Design review of the part built by this model. Coordinates are the model's own, in mm. A direction names the side the tool comes from. Round coordinates to 2 decimals unless told otherwise and drop trailing zeros. Loops run counter-clockwise (first coordinate to the right, second up) from the corner with the lowest first, then second, coordinate; pieces in that order, holes last. Notation, with made-up numbers: (-0.75, 2) - (45.25, 2) arc R21 ccw to (45.25, 40) - close; hole circle Ø4 at (23, 19.5). An arc over 180 degrees is marked (long way). Return JSON: item names as keys, results as strings. Group by question number.
(1) We need section D-D, the plane x = 20.5. Write out the cut boundary in (y, z).
(2) Clearance check with flat-ended pins moving along their axes: pin 1 (2 mm diameter, centred on x = -41.5, y = 46, fed in from +Z); pin 2 (1 mm diameter, centred on y = 9.5, z = 18.5, fed in from -X); pin 3 (0.6 mm diameter, centred on y = 21, z = 18.5, fed in from -X). State where each tip first meets the part, or that it passes through.
(3) We need section C-C, the plane x = -4. Write out the cut boundary in (y, z), and give its area (3 significant figures).
(4) We need section A-A, the plane z = 0. Write out the cut boundary in (x, y).
(5) The part is to be moulded in two halves that separate along Y. For faces 4 (the flat face through (-6, 85, 0)), 5 (the flat face through (-7, 83, 1)), 6 (the flat face through (-15, 42, -19.3)), 7 (the flat face through (3.201, 23, 18)), say which applies: pulls with the +Y half, pulls with the -Y half, needs draft (parallel to the pull), parting line crosses it, or undercut.
(6) We need section B-B, the plane y = 19. Write out the cut boundary in (x, z), and give its area (3 significant figures).
(7) For faces 1 (the cylindrical face through (30.597, 40.919, -0.383)), 2 (the flat face through (-40.799, 41, 0)), 3 (the flat face through (-2, 13, 18)), list the 3-axis set-ups (+Z, -Z, +X, -X, +Y, -Y) from which the entire face can be reached by the end or side of a thin tool; tool diameter is ignored.
(8) Wall thickness on L1, parallel to Y at x = 27, z = -1.5; L2, parallel to Z at x = 4.5, y = 19; L3, parallel to X at y = 32, z = 0.5: over which ranges is each line inside the solid? List them lowest first. Write a range as [from, to].
Autodesk Inventor part; units mm, degrees
ref_plane "Work Plane1" through (0, 85, 0) normal (0, 1, 0) x (1, 0, 0)
ref_plane "Work Plane2" through (-42.6987, 0, 19.3) normal (0, -1, 0) x (1, 0, 0)
ref_plane "YZ Plane" through (0, 0, 0) normal (1, 0, 0) x (0, 1, 0)
sketch "Sketch1" plane through (0, 0, 0) normal (0, 1, 0) x (-1, 0, 0)
  line L0 (40.7987, 17.4) -> (40.7987, -17.4)
  line L1 (40.7987, -17.4) -> (-13.2013, -17.4)
  arc A0 (-13.2013, 17.4) -> (-13.2013, -17.4) centre (-13.2013, 0) ccw
  line L2 (-13.2013, 17.4) -> (40.7987, 17.4)
  line L3 (42.6987, -19.3) -> (42.6987, 19.3)
  line L4 (42.6987, 19.3) -> (-13.2013, 19.3)
  arc A1 (-13.2013, 19.3) -> (-13.2013, -19.3) centre (-13.2013, 0) ccw
  line L5 (-13.2013, -19.3) -> (42.6987, -19.3)
  point P0 (0, 0)
  point P1 (-13.2013, 0)
  point P2 (0, 0)
  point P3 (-12.8411, -36.7096)
  point P4 (-12.8411, -7.716)
  point P5 (-24.0253, -72.4098)
  dimension "d156" = 1.9
  dimension "d157" = 1.9
  dimension "d158" = 1.9
  dimension "d159" = 1.9
  dimension "d160" = 54
extrude "Extrusion1" add sketch "Sketch1" along normal blind 83
ref_plane "Work Plane1" through (0, 85, 0) normal (0, 1, 0) x (1, 0, 0)
sketch "Sketch2" plane through (0, 85, 0) normal (0, 1, 0) x (1, 0, 0)
  line L0 (-42.6987, 19.3) -> (-42.6987, -19.3)
  line L1 (-42.6987, -19.3) -> (13.2013, -19.3)
  arc A0 (13.2013, -19.3) -> (13.2013, 19.3) centre (13.2013, 0) ccw
  line L2 (13.2013, 19.3) -> (-42.6987, 19.3)
  line L3 (-42.6987, 19.3) -> (-42.6987, -19.3)
  line L4 (-42.6987, -19.3) -> (13.2013, -19.3)
  arc A1 (13.2013, -19.3) -> (13.2013, 19.3) centre (13.2013, 0) ccw
  point P0 (0, 0)
  point P1 (14.0497, 95.3418)
  point P2 (14.0497, 124.3354)
  point P3 (2.8654, 59.6417)
  dimension "d163" = 38.6
  dimension "d165" = 19.3
  dimension "d166" = 0
  dimension "d167" = 0
  dimension "d168" = 0
extrude "Extrusion2" add sketch "Sketch2" against normal up to surface (2 mm away)
ref_plane "Work Plane2" through (-42.6987, 0, 19.3) normal (0, -1, 0) x (1, 0, 0)
sketch "Sketch35" plane through (-42.6987, 0, 19.3) normal (0, -1, 0) x (1, 0, 0)
  line L0 (0, 0) -> (0, -38.6)
  line L1 (0, -38.6) -> (55.9, -38.6)
  arc A0 (55.9, -38.6) -> (55.9, 0) centre (55.9, -19.3) ccw
  line L2 (55.9, 0) -> (0, 0)
  line L3 (0, 0) -> (55.9, 0)
  arc A1 (55.9, -38.6) -> (55.9, 0) centre (55.9, -19.3) ccw
  line L4 (0, -38.6) -> (0, 0)
  point P0 (17.1629, -27.1873)
  point P1 (30.3642, -27.1873)
  point P2 (17.1629, -27.1873)
  point P3 (14.0497, 95.3418)
  point P4 (14.0497, 124.3354)
  point P5 (2.8654, 59.6417)
  dimension "d132" = 19.3
  dimension "d133" = 0
  dimension "d162" = 0
extrude "Extrusion24" add sketch "Sketch35" along normal blind 2
sketch "Sketch37" plane through (-42.6987, 85, 19.3) normal (0, 0, 1) x (1, 0, 0)
  line L0 (35.9, -85) -> (0, -85)
  line L1 (0, -85) -> (0, -2)
  line L2 (0, -2) -> (35.9, -2)
  line L3 (35.9, -2) -> (35.9, -85)
  line L4 (55.9, -85) -> (1.9, -85)
  line L5 (55.9, -2) -> (1.9, -2)
  line L6 (0, 0) -> (0, -87)
  line L7 (55.9, -87) -> (55.9, 0)
  point P0 (42.6987, -85)
  dimension "d143" = 0
  dimension "d144" = 0
  dimension "d145" = 0
  dimension "d146" = 20
extrude "Extrusion26" cut sketch "Sketch37" against normal up to surface (1.9 mm away) contours L0 L1 L2 L3
sketch "Sketch38" plane through (-42.6987, 85, 19.3) normal (0, 0, 1) x (1, 0, 0)
  line L0 (35.9, -85) -> (35.9, -2)
  line L1 (45.9, -72) -> (35.9, -72)
  line L2 (35.9, -72) -> (35.9, -52)
  line L3 (35.9, -52) -> (45.9, -52)
  line L4 (45.9, -52) -> (45.9, -72)
  line L5 (55.9, -87) -> (0, -87)
  point P0 (42.6987, -85)
  point P1 (35.9, -72)
  dimension "d149" = 20
  dimension "d150" = 10
  dimension "d151" = 15
extrude "Extrusion27" cut sketch "Sketch38" against normal up to surface (1.9 mm away)
properties part number "víko"
Solutions:
{
 "1": {"outline": "(-2, -17.87) - (85, -17.87) - (85, 17.87) - (-2, 17.87) - close; hole (0, -15.8) - (83, -15.8) - (83, 15.8) - (0, 15.8) - close"},
 "2": {"pin 1": "z = 17.4", "pin 2": "x = -6.8", "pin 3": "x = 3.2"},
 "3": {"outline": "(-2, -19.3) - (85, -19.3) - (85, 19.3) - (33, 19.3) - (33, 17.4) - (83, 17.4) - (83, -17.4) - (0, -17.4) - (0, 17.4) - (13, 17.4) - (13, 19.3) - (-2, 19.3) - close", "area": "432 mm^2"},
 "4": {"outline": "(-42.7, -2) - (32.5, -2) - (32.5, 85) - (-42.7, 85) - close; hole (-40.8, 0) - (30.6, 0) - (30.6, 83) - (-40.8, 83) - close"},
 "5": {"face 4": "pulls with the +Y half", "face 5": "undercut", "face 6": "needs draft", "face 7": "undercut"},
 "6": {"outline": "(-42.7, -19.3) - (13.2, -19.3) arc R19.3 ccw to (13.2, 19.3) - (3.2, 19.3) - (3.2, 17.4) - (13.2, 17.4) arc R17.4 cw to (13.2, -17.4) - (-40.8, -17.4) - (-40.8, 17.4) - (-42.7, 17.4) - close", "area": "301 mm^2"},
 "7": {"face 1": "none", "face 2": "+Z", "face 3": "+Z, -X"},
 "8": {"L1": "[-2, 0], [83, 85]", "L2": "[-19.3, -17.4], [17.4, 19.3]", "L3": "[-42.7, -40.8], [30.59, 32.49]"}
}
